Read the model definition and answer for the solid it produces. Units are mm, in the model's axes. Coordinates: 2 decimals unless noted, no trailing zeros. Order: outer loops, then holes, each group sorted by start corner. A loop starts at its lowest first (then second) coordinate and runs counter-clockwise, first axis right, second up.
```python
from build123d import *

# Parameters (mm, degrees)
BOSS_EXTRUDE1_DEPTH = 3.175
SKETCH2_R           = 3.175
CUT_EXTRUDE1_DEPTH  = 34.531039724
LPATTERN1_COUNT     = 2
LPATTERN1_PITCH     = 24
LPATTERN1_COL_COUNT = 2
LPATTERN1_COL_PITCH = 24


with BuildPart() as part:
    # Sketch1 → Boss-Extrude1 (new body)
    with BuildSketch(Plane.XY):
        with BuildLine():
            Line((-9.5, -22.5), (-9.5, 22.5))
            ThreePointArc((-9.5, 22.5), (0, 32), (9.5, 22.5))
            Line((9.5, 22.5), (9.5, -22.5))
            ThreePointArc((9.5, -22.5), (0, -32), (-9.5, -22.5))
        make_face()
    extrude(amount=BOSS_EXTRUDE1_DEPTH)

    # Sketch2 → Cut-Extrude1 (cut, through all)
    with BuildSketch(Plane.XY.offset(3.175)):
        Circle(SKETCH2_R)
    cut_extrude1 = extrude(amount=-CUT_EXTRUDE1_DEPTH, mode=Mode.SUBTRACT)

    # LPattern1: Cut-Extrude1 ×2
    with Locations(*[(0, i * LPATTERN1_PITCH, 0) for i in range(1, LPATTERN1_COUNT)]):
        add(cut_extrude1, mode=Mode.SUBTRACT)

    # LPattern1 col: Cut-Extrude1 ×2
    with Locations(*[(0, -i * LPATTERN1_COL_PITCH, 0) for i in range(1, LPATTERN1_COL_COUNT)]):
        add(cut_extrude1, mode=Mode.SUBTRACT)


solid = part.part
```
1) A flat-ended cylindrical pin translates along its axis: pin 1 Ø4 at (x, y) = (0, 24) entering from -Z. Find the tip coordinate at first contact, or state that the pin passes through.
A:
pin 1: passes through
2) A cutting plane is placed at D-D, the plane y = -24. Determine the outline of the cut face in (x, z) (3 decimals), and give its area (3 significant figures).
A:
outline: (-9.381, 0) - (-3.175, 0) - (-3.175, 3.175) - (-9.381, 3.175) - close; (3.175, 0) - (9.381, 0) - (9.381, 3.175) - (3.175, 3.175) - close
area: 39.4 mm2
3) A cutting plane is placed at A-A, the plane x = 0. Determine the outline of the cut face in (y, z) (3 decimals).
A:
outline: (-32, 0) - (-27.175, 0) - (-27.175, 3.175) - (-32, 3.175) - close; (-20.825, 0) - (-3.175, 0) - (-3.175, 3.175) - (-20.825, 3.175) - close; (3.175, 0) - (20.825, 0) - (20.825, 3.175) - (3.175, 3.175) - close; (27.175, 0) - (32, 0) - (32, 3.175) - (27.175, 3.175) - close
4) Straight lines are drawn through the part: line 1 (Y direction, x = 0, z = 0.95) (3 decimals); line 2 (Y direction, x = -2.5, z = 1); line 3 (X direction, y = 25.5, z = 2.35). For each, find the intervals that lie inside material, in ascending order.
A:
line 1: y = -32 to -27.175, -20.825 to -3.175, 3.175 to 20.825, 27.175 to 32
line 2: y = -31.67 to -25.96, -22.04 to -1.96, 1.96 to 22.04, 25.96 to 31.67
line 3: x = -9.01 to -2.8, 2.8 to 9.01
5) A cutting plane is placed at B-B, the plane z = 1.25. Determine the outline of the cut face in (x, y) (3 decimals).
A:
outline: (-9.5, -22.5) arc R9.5 ccw to (9.5, -22.5) - (9.5, 22.5) arc R9.5 ccw to (-9.5, 22.5) - close; hole circle Ø6.35 at (0, -24); hole circle Ø6.35 at (0, 0); hole circle Ø6.35 at (0, 24)
6) A cutting plane is placed at C-C, the plane y = 0. Determine the outline of the cut face in (x, z) (3 decimals), and give its area (3 significant figures).
A:
outline: (-9.5, 0) - (-3.175, 0) - (-3.175, 3.175) - (-9.5, 3.175) - close; (3.175, 0) - (9.5, 0) - (9.5, 3.175) - (3.175, 3.175) - close
area: 40.2 mm2
7) Determine the mould class of faces 1 (the cylindrical face through (-0.69, -3.1, 1.61)), 2 (the flat face through (-9.5, 0, 2)), 3 (the flat face through (4, 0, 3.175)) for opening direction X: pulls with the +X half, pulls with the -X half, needs draft (parallel to the pull), parting line crosses it, or undercut.
A:
face 1: undercut
face 2: pulls with the -X half
face 3: needs draft
